```python
from build123d import *

# Parameters (mm, degrees)
SKETCH_1_R          = 6.8
EXTRUDE_1_DEPTH     = 10
SKETCH_3_W          = 5.484573778
SKETCH_3_H          = 13.374261712
EXTRUDE_2_DEPTH     = 10
SKETCH_2_R          = 5.35
CUT_EXTRUDE_1_DEPTH = 10
SKETCH_4_W          = 2.844022018
SKETCH_4_H          = 17.569991778
CUT_EXTRUDE_2_DEPTH = 10
SKETCH_5_R          = 1.3
CUT_EXTRUDE_3_DEPTH = 10


with BuildPart() as part:
    # 草图1 → 凸台-拉伸1 (new body)
    with BuildSketch(Plane(origin=(0, 0, 0), x_dir=(1, 0, 0), z_dir=(0, 1, 0))):
        with Locations(Location((0, 0, 0), (0, 0, 270))):
            Circle(SKETCH_1_R)
    extrude(amount=EXTRUDE_1_DEPTH)

    # 草图3 → 凸台-拉伸2 (add)
    with BuildSketch(Plane(origin=(0, 0, 0), x_dir=(1, 0, 0), z_dir=(0, 1, 0))):
        with Locations((0, -6.642082697)):
            Rectangle(SKETCH_3_W, SKETCH_3_H)
    extrude(amount=EXTRUDE_2_DEPTH)

    # 草图2 → 切除-拉伸1 (cut)
    with BuildSketch(Plane(origin=(0, 10, 0), x_dir=(1, 0, 0), z_dir=(0, 1, 0))):
        with Locations(Location((0, 0, 0), (0, 0, 270))):
            Circle(SKETCH_2_R)
    extrude(amount=-CUT_EXTRUDE_1_DEPTH, mode=Mode.SUBTRACT)

    # 草图4 → 切除-拉伸2 (cut)
    with BuildSketch(Plane(origin=(0, 0, 0), x_dir=(1, 0, 0), z_dir=(0, 1, 0))):
        with Locations((0, -13.329213553)):
            Rectangle(SKETCH_4_W, SKETCH_4_H)
    extrude(amount=CUT_EXTRUDE_2_DEPTH, mode=Mode.SUBTRACT)

    # 草图5 → 切除-拉伸3 (cut)
    with BuildSketch(Plane(origin=(2.742286889, 0, 0), x_dir=(0, 0, -1), z_dir=(1, 0, 0))):
        with Locations((-9.775871094, 5)):
            Circle(SKETCH_5_R)
    extrude(amount=-CUT_EXTRUDE_3_DEPTH, mode=Mode.SUBTRACT)


solid = part.part
```
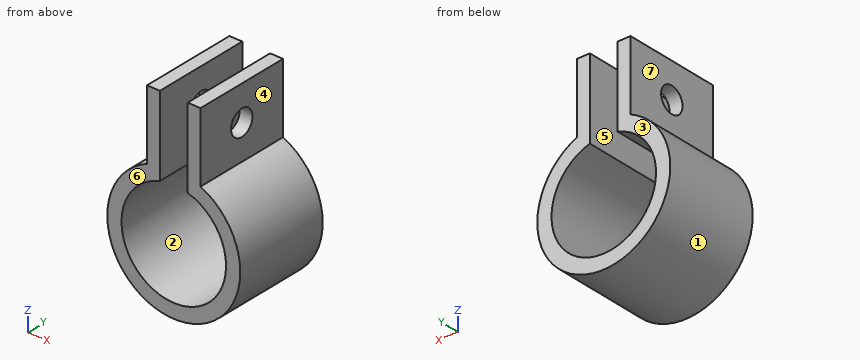
Verification items for the finished model (mm, model axes). Face numbers are marked on the shaded views. A direction names the side the tool comes from. Round coordinates to 2 decimals unless told otherwise and drop trailing zeros. Write each loop counter-clockwise with the first axis right and the second up, starting at its lowest first coordinate (ties: lowest second). Pieces come first, ordered by that corner, then holes.
1. Gauge pin test, flat ends, axial feed: P1, Ø1.6, axis at y = 5, z = 9.78, coming from the -X side; P2, Ø3, axis at y = 5, z = 9.78, coming from the -X side; P3, Ø3.5, axis at y = 3, z = 11, coming from the +X side; P4, Ø5, axis at x = 1, y = 1.5, coming from the -Z side. Record the tip position at first contact, or that the pin passes through.
2. Access from +Z, -Z, +X, -X, +Y, -Y to the whole of each face (thin tool, end or side, straight path). Record for the marked faces 4, 5, 6 and 7.
3. Section check D-D on y = 3. Enter the section's corners in (x, z).
4. Section check A-A on y = 5. Enter the section's corners in (x, z), plus the area to 3 significant figures.
5. Scan lines: L1, parallel to X at y = 3, z = 11; L2, parallel to X at y = 4.25, z = 0; L3, parallel to Z at x = -1, y = 3.75. Record each from-to range of solid material in increasing order.
6. Section check C-C on x = -2. Enter the section's corners in (y, z).
7. Draft check along X on the marked faces 1, 2 and 3. Enter one of: +X half, -X half, draft (parallel to the pull), parting line (faces both ways), or undercut.
8. Section check B-B on z = 0. Enter the section's corners in (x, y).
Answer:
1. P1: passes through
1. P2: stops at x = -2.74
1. P3: stops at x = 2.74
1. P4: stops at z = -6.8
2. face 4: +Z, +X, +Y, -Y
2. face 5: +Z, +Y, -Y
2. face 6: +Z, -Z, +X, -X, -Y
2. face 7: +Z, -X, +Y, -Y
3. outline: (-2.74, 6.22) arc R6.8 ccw (long way) to (2.74, 6.22) - (2.74, 13.33) - (1.42, 13.33) - (1.42, 5.16) arc R5.35 cw (long way) to (-1.42, 5.16) - (-1.42, 13.33) - (-2.74, 13.33) - close
4. outline: (-2.74, 6.22) arc R6.8 ccw (long way) to (2.74, 6.22) - (2.74, 8.48) - (1.42, 8.48) - (1.42, 5.16) arc R5.35 cw (long way) to (-1.42, 5.16) - (-1.42, 8.48) - (-2.74, 8.48) - close; (-2.74, 11.08) - (-1.42, 11.08) - (-1.42, 13.33) - (-2.74, 13.33) - close; (1.42, 11.08) - (2.74, 11.08) - (2.74, 13.33) - (1.42, 13.33) - close
4. area: 62.5 mm2
5. L1: x = -2.74 to -1.42, 1.42 to 2.74
5. L2: x = -6.8 to -5.35, 5.35 to 6.8
5. L3: z = -6.73 to -5.26
6. outline: (0, -6.5) - (10, -6.5) - (10, -4.96) - (0, -4.96) - close; (0, 4.96) - (10, 4.96) - (10, 13.33) - (0, 13.33) - close; hole circle Ø2.6 at (5, 9.78)
7. face 1: parting line
7. face 2: undercut
7. face 3: draft
8. outline: (-6.8, 0) - (-5.35, 0) - (-5.35, 10) - (-6.8, 10) - close; (5.35, 0) - (6.8, 0) - (6.8, 10) - (5.35, 10) - close
